Source: CAD feature listing. Evaluate the final solid. Frame: model axes, mm. A direction names the side the tool comes from. Give positions to 0.01 mm unless a question says otherwise; leave off trailing zeros. Write each loop counter-clockwise with the first axis right and the second up, starting at its lowest first coordinate (ties: lowest second). Pieces come first, ordered by that corner, then holes.
```python
from build123d import *

# Parameters (mm, degrees)
F1_DEPTH = 2.54
F2_DEPTH = 5.08


with BuildPart() as f1:
    # F0 (on Front) → F1 (new body)
    with BuildSketch(Plane.XZ):
        with BuildLine():
            ThreePointArc((50.034948, -30.582519), (56.448624, -15.885194), (58.641167, 0))
            ThreePointArc((58.641167, 0), (53.846731, 23.223178), (40.2474, 42.648954))
            add(Edge.make_bspline(
                [(16.570685, 26.408125), (23.263536, 32.695353), (30.564828, 38.576946), (40.2474, 42.648954)],
                knots=[0, 0, 0, 0, 28.711519, 28.711519, 28.711519, 28.711519], degree=3))
            add(Edge.make_bspline(
                [(16.570685, 26.408125), (29.209305, 8.924421), (43.342095, -11.112408), (50.034948, -30.582519)],
                knots=[0, 0, 0, 0, 66.08926, 66.08926, 66.08926, 66.08926], degree=3))
        make_face()
        with BuildLine():
            add(Edge.make_bspline(
                [(16.570685, 26.408125), (23.263536, 32.695353), (30.564828, 38.576946), (40.2474, 42.648954)],
                knots=[0, 0, 0, 0, 28.711519, 28.711519, 28.711519, 28.711519], degree=3))
            ThreePointArc((40.2474, 42.648954), (35.461347, 46.704169), (30.269499, 50.224933))
            add(Edge.make_bspline(
                [(30.269499, 50.224933), (20.221332, 50.542954), (8.458137, 47.500748), (0, 41.41634)],
                knots=[0, 0, 0, 0, 31.525131, 31.525131, 31.525131, 31.525131], degree=3))
            add(Edge.make_bspline(
                [(0, 41.41634), (-9.795095, 47.500748), (-20.138593, 49.326073), (-29.225386, 50.839584)],
                knots=[0, 0, 0, 0, 30.707014, 30.707014, 30.707014, 30.707014], degree=3))
            ThreePointArc((-29.225386, 50.839584), (-35.011661, 47.042216), (-40.310237, 42.589568))
            Line((-40.310237, 42.589568), (-38.189009, 41.821968))
            add(Edge.make_bspline(
                [(-38.189009, 41.821968), (-28.453952, 38.779758), (-22.369543, 32.492537), (-15.473878, 26.205312)],
                knots=[0, 0, 0, 0, 27.565505, 27.565505, 27.565505, 27.565505], degree=3))
            add(Edge.make_bspline(
                [(-15.473878, 26.205312), (-28.859582, 6.735198), (-44.273421, -11.112408), (-45.89593, -33.82754)],
                knots=[0, 0, 0, 0, 67.301148, 67.301148, 67.301148, 67.301148], degree=3))
            Line((-45.89593, -33.82754), (-46.222024, -36.087546))
            ThreePointArc((-46.222024, -36.087546), (-42.685571, -40.208562), (-38.783069, -43.98477))
            Line((-38.783069, -43.98477), (-38.797453, -42.751342))
            add(Edge.make_bspline(
                [(-38.797453, -42.751342), (-40.014334, -22.875601), (-19.935779, -8.678642), (0, 9.980217)],
                knots=[0, 0, 0, 0, 65.466477, 65.466477, 65.466477, 65.466477], degree=3))
            add(Edge.make_bspline(
                [(0, 9.980217), (21.032587, 0), (36.810137, -25.684895), (41.660637, -41.269574)],
                knots=[0, 0, 0, 0, 66.046573, 66.046573, 66.046573, 66.046573], degree=3))
            ThreePointArc((41.660637, -41.269574), (46.158134, -36.169229), (50.034948, -30.582519))
            add(Edge.make_bspline(
                [(16.570685, 26.408125), (29.209305, 8.924421), (43.342095, -11.112408), (50.034948, -30.582519)],
                knots=[0, 0, 0, 0, 66.08926, 66.08926, 66.08926, 66.08926], degree=3))
        make_face()
        with BuildLine():
            add(Edge.make_bspline(
                [(30.269499, 50.224933), (20.221332, 50.542954), (8.458137, 47.500748), (0, 41.41634)],
                knots=[0, 0, 0, 0, 31.525131, 31.525131, 31.525131, 31.525131], degree=3))
            ThreePointArc((30.269499, 50.224933), (0.605799, 58.638038), (-29.225386, 50.839584))
            add(Edge.make_bspline(
                [(0, 41.41634), (-9.795095, 47.500748), (-20.138593, 49.326073), (-29.225386, 50.839584)],
                knots=[0, 0, 0, 0, 30.707014, 30.707014, 30.707014, 30.707014], degree=3))
        make_face()
        with BuildLine():
            ThreePointArc((-38.783069, -43.98477), (1.978174, -58.607792), (41.660637, -41.269574))
            add(Edge.make_bspline(
                [(0, 9.980217), (21.032587, 0), (36.810137, -25.684895), (41.660637, -41.269574)],
                knots=[0, 0, 0, 0, 66.046573, 66.046573, 66.046573, 66.046573], degree=3))
            add(Edge.make_bspline(
                [(-38.797453, -42.751342), (-40.014334, -22.875601), (-19.935779, -8.678642), (0, 9.980217)],
                knots=[0, 0, 0, 0, 65.466477, 65.466477, 65.466477, 65.466477], degree=3))
            Line((-38.797453, -42.751342), (-38.783069, -43.98477))
        make_face()
        with BuildLine():
            Line((-38.189009, 41.821968), (-40.310237, 42.589568))
            ThreePointArc((-40.310237, 42.589568), (-58.476321, 4.393902), (-46.222024, -36.087546))
            Line((-46.222024, -36.087546), (-45.89593, -33.82754))
            add(Edge.make_bspline(
                [(-15.473878, 26.205312), (-28.859582, 6.735198), (-44.273421, -11.112408), (-45.89593, -33.82754)],
                knots=[0, 0, 0, 0, 67.301148, 67.301148, 67.301148, 67.301148], degree=3))
            add(Edge.make_bspline(
                [(-38.189009, 41.821968), (-28.453952, 38.779758), (-22.369543, 32.492537), (-15.473878, 26.205312)],
                knots=[0, 0, 0, 0, 27.565505, 27.565505, 27.565505, 27.565505], degree=3))
        make_face()
    extrude(amount=F1_DEPTH)

    # F0 (on Front) → F2 (join)
    with BuildSketch(Plane.XZ):
        with BuildLine():
            add(Edge.make_bspline(
                [(16.570685, 26.408125), (23.263536, 32.695353), (30.564828, 38.576946), (40.2474, 42.648954)],
                knots=[0, 0, 0, 0, 28.711519, 28.711519, 28.711519, 28.711519], degree=3))
            ThreePointArc((40.2474, 42.648954), (35.461347, 46.704169), (30.269499, 50.224933))
            add(Edge.make_bspline(
                [(30.269499, 50.224933), (20.221332, 50.542954), (8.458137, 47.500748), (0, 41.41634)],
                knots=[0, 0, 0, 0, 31.525131, 31.525131, 31.525131, 31.525131], degree=3))
            add(Edge.make_bspline(
                [(0, 41.41634), (-9.795095, 47.500748), (-20.138593, 49.326073), (-29.225386, 50.839584)],
                knots=[0, 0, 0, 0, 30.707014, 30.707014, 30.707014, 30.707014], degree=3))
            ThreePointArc((-29.225386, 50.839584), (-35.011661, 47.042216), (-40.310237, 42.589568))
            Line((-40.310237, 42.589568), (-38.189009, 41.821968))
            add(Edge.make_bspline(
                [(-38.189009, 41.821968), (-28.453952, 38.779758), (-22.369543, 32.492537), (-15.473878, 26.205312)],
                knots=[0, 0, 0, 0, 27.565505, 27.565505, 27.565505, 27.565505], degree=3))
            add(Edge.make_bspline(
                [(-15.473878, 26.205312), (-28.859582, 6.735198), (-44.273421, -11.112408), (-45.89593, -33.82754)],
                knots=[0, 0, 0, 0, 67.301148, 67.301148, 67.301148, 67.301148], degree=3))
            Line((-45.89593, -33.82754), (-46.222024, -36.087546))
            ThreePointArc((-46.222024, -36.087546), (-42.685571, -40.208562), (-38.783069, -43.98477))
            Line((-38.783069, -43.98477), (-38.797453, -42.751342))
            add(Edge.make_bspline(
                [(-38.797453, -42.751342), (-40.014334, -22.875601), (-19.935779, -8.678642), (0, 9.980217)],
                knots=[0, 0, 0, 0, 65.466477, 65.466477, 65.466477, 65.466477], degree=3))
            add(Edge.make_bspline(
                [(0, 9.980217), (21.032587, 0), (36.810137, -25.684895), (41.660637, -41.269574)],
                knots=[0, 0, 0, 0, 66.046573, 66.046573, 66.046573, 66.046573], degree=3))
            ThreePointArc((41.660637, -41.269574), (46.158134, -36.169229), (50.034948, -30.582519))
            add(Edge.make_bspline(
                [(16.570685, 26.408125), (29.209305, 8.924421), (43.342095, -11.112408), (50.034948, -30.582519)],
                knots=[0, 0, 0, 0, 66.08926, 66.08926, 66.08926, 66.08926], degree=3))
        make_face()
    extrude(amount=F2_DEPTH)


solid = f1.part
```
1. Access query for faces 5 (the flat face through (42, -2.54, 15)), 6 (the flat face through (-42, -2.54, 13)), 7 (the flat face through (1, -5.08, 15)). Directions: +Z, -Z, +X, -X, +Y, -Y. A direction counts if a zero-diameter tool reaches every point of the face in a straight line with its end or side. Return the directions, or none.
2. Line query: probe 1 along Y at (x, z) = (-52.5, -8.5); probe 2 along Z at (x, y) = (-28, -3.15); probe 3 along X at (y, z) = (-3.2, -28.5). Output: solid intervals per line, ascending.
3. Section query A-A (y = -1.55). Return loops of the section in (x, z).
4. Pin query (flat end, axial travel): P1, Ø8, axis at x = 26.5, z = -25.5, coming from the -Y side; P2, Ø1, axis at y = -4, z = 9.5, coming from the -X side; P3, Ø3, axis at x = -26.5, y = -0.5, coming from the -Z side. Return the tip coordinate at first contact, or that it passes through.
5. Pull-direction query (X, two-part tool) for faces 1 (the flat face through (-1, 0, 1)), 2 (the flat face through (0, -2.54, 52)), 3 (the cylindrical face through (53.978, -1.252, 22.916)), 4 (the flat face through (1, -2.54, -31)); classes: pulls with the +X half, pulls with the -X half, needs draft (parallel to the pull), parting line crosses it, or undercut.
The answers:
1. face 5: +X, -Y
1. face 6: -X, -Y
1. face 7: +Z, -Z, +X, -X, -Y
2. probe 1: y = -2.54 to 0
2. probe 2: z = -16.7 to 8.42, 36.84 to 50.63
2. probe 3: x = -45.26 to -35.94, 36.28 to 49.29
3. outline: (-46.22, -36.09) arc R58.64 ccw to (-38.78, -43.98) arc R58.64 ccw to (41.66, -41.27) arc R58.64 ccw to (50.03, -30.58) arc R58.64 ccw to (58.64, 0) arc R58.64 ccw to (40.25, 42.65) arc R58.64 ccw to (30.27, 50.22) arc R58.64 ccw to (-29.23, 50.84) arc R58.64 ccw to (-40.31, 42.59) arc R58.64 ccw to start
4. P1: stops at y = -2.54
4. P2: stops at x = -27.6
4. P3: stops at z = -53.05
5. face 1: needs draft
5. face 2: undercut
5. face 3: pulls with the +X half
5. face 4: undercut
